Input: part model. Units: mm. Frame: model coordinates. A direction names the side the tool comes from. Round coordinates to 2 decimals unless told otherwise and drop trailing zeros. Loops run counter-clockwise (first coordinate to the right, second up) from the corner with the lowest first, then second, coordinate; pieces in that order, holes last. Notation, with made-up numbers: (65, -14.75) - (109, -14.75) arc R13 ccw to (109, 0.25) - close; hole circle Ø10 at (26.25, 13). An arc over 180 degrees is marked (long way). Use CSV: the item, a comma, the result in double quotes. Start each with the question number.
1. Pin query (flat end, axial travel): P1, Ø5, axis at y = 3.5, z = -101.5, coming from the -X side; P2, Ø2, axis at x = 11, y = 19.5, coming from the -Z side; P3, Ø4, axis at x = 11.5, y = 15.5, coming from the +Z side. Return the tip coordinate at first contact, or that it passes through.
2. Cut plane C-C (z = -21.5). Return loops of the section in (x, y) (3 decimals).
3. Cut plane B-B (z = -69.7). Return loops of the section in (x, y), and give its area (3 significant figures).
4. Access query for faces 1 (the flat face through (0, 9, -13)), 2 (the flat face through (24, 20, -85.5)), 3 (the cylindrical face through (46.55, 5.46, -69.59)), 4 (the flat face through (21.5, 15, -95)), 5 (the flat face through (0, 9, -5)). Directions: +Z, -Z, +X, -X, +Y, -Y. A direction counts if a zero-diameter tool reaches every point of the face in a straight line with its end or side. Return the directions, or none.
5. Cut plane A-A (z = -53). Return loops of the section in (x, y).
6. Pull-direction query (Y, two-part tool) for faces 6 (the flat face through (48.2, 6, -102)), 7 (the flat face through (0, 9, -25)), 8 (the flat face through (54, 11.8, -102)); classes: +Y half, -Y half, draft (parallel to the pull), parting line (faces both ways), or undercut.
7. Material intervals for probe 1 along Z at (x, y) = (24, 21.75); probe 2 along X at (y, z) = (17.5, -88); probe 3 along X at (y, z) = (6.95, -69.7), sorted ascending. Write a range as from..to.
```python
from build123d import *

# Parameters (mm, degrees)
EXTRUDE_1_DEPTH     = 60
SHELL_1_T           = -2.5
SKETCH_3_R          = 2.25
EXTRUDE_3_DEPTH     = 4
CUT_EXTRUDE_1_DEPTH = 118.856904762
SKETCH_5_R          = 2.2
EXTRUDE_4_DEPTH     = 6
SKETCH_7_W          = 42
SKETCH_7_H          = 12
CUT_EXTRUDE_3_DEPTH = 2.5
SKETCH_8_W          = 10.4
SKETCH_8_H          = 12
EXTRUDE_5_DEPTH     = 2.5
SKETCH_9_W          = 7
SKETCH_9_H          = 7
SKETCH_9_R          = 2.2
EXTRUDE_6_DEPTH     = 8
SKETCH_10_R         = 2.2
EXTRUDE_7_DEPTH     = 5
EXTRUDE_8_DEPTH     = 4
EXTRUDE_10_DEPTH    = 4
SKETCH_14_R         = 3
CUT_EXTRUDE_4_DEPTH = 119.584358159
SKETCH_15_W         = 16
SKETCH_15_H         = 2
CUT_EXTRUDE_5_DEPTH = 1.4
CUT_EXTRUDE_6_REACH = 121.933
SKETCH_16_W         = 12
SKETCH_16_H         = 14
SKETCH_17_W         = 12
SKETCH_17_H         = 14
EXTRUDE_14_DEPTH    = 2
EXTRUDE_15_REACH    = 120.238
SKETCH_18_W         = 3.2
SKETCH_18_H         = 3.2
SKETCH_19_W         = 5.75
SKETCH_19_H         = 10.4
CUT_EXTRUDE_7_DEPTH = 4
SKETCH_20_W         = 55
SKETCH_20_H         = 3
CUT_EXTRUDE_8_DEPTH = 0.5
SKETCH_22_R         = 2.2
EXTRUDE_17_DEPTH    = 5
SKETCH_23_R         = 2.897416755
EXTRUDE_18_DEPTH    = 2
FILLET_1_R          = 2
CUT_EXTRUDE_9_REACH = 127.999
SKETCH_25_W         = 5.8
SKETCH_25_H         = 5.8
SKETCH_26_W         = 5.8
SKETCH_26_H         = 4
EXTRUDE_19_DEPTH    = 1
SKETCH_27_W         = 10
SKETCH_27_H         = 4
EXTRUDE_20_DEPTH    = 2
SKETCH_28_W         = 11.8
SKETCH_28_H         = 11.8
SKETCH_28_W_2       = 5.8
SKETCH_28_H_2       = 5.8
EXTRUDE_23_DEPTH    = 4.5


with BuildPart() as part:
    # 草图1 → 凸台-拉伸1 (new body)
    with BuildSketch(Plane(origin=(0, 0, 0), x_dir=(0, 0, -1), z_dir=(1, 0, 0))):
        Polygon((0, 0), (100, 0), (100, 28), (0, 17), align=None)
    extrude(amount=EXTRUDE_1_DEPTH)

    # 抽壳1
    shell_1_openings = [part.faces().sort_by_distance(p)[0] for p in [
        (30, 22.5, -50),
    ]]
    offset(amount=SHELL_1_T, openings=shell_1_openings, kind=Kind.INTERSECTION)

    # 草图3 → 凸台-拉伸3 (add)
    # profile 1 of 2: a face of its own
    with BuildSketch(Plane(origin=(0, 2.5, 0), x_dir=(1, 0, 0), z_dir=(0, 1, 0))):
        with BuildLine():
            Line((2.5, 97.5), (2.5, 85.75))
            ThreePointArc((2.5, 85.75), (6.685854123, 84.442437632), (9.25, 88))
            Line((9.25, 88), (9.25, 97.5))
            Line((9.25, 97.5), (2.5, 97.5))
        make_face()
        with Locations(Location((5.5, 88, 0), (0, 0, 270))):
            Circle(SKETCH_3_R, mode=Mode.SUBTRACT)
    # profile 2 of 2: a face of its own
    with BuildSketch(Plane(origin=(0, 2.5, 0), x_dir=(1, 0, 0), z_dir=(0, 1, 0))):
        with BuildLine():
            Line((16.75, 88), (16.75, 97.5))
            Line((16.75, 97.5), (24.25, 97.5))
            Line((24.25, 97.5), (24.25, 88))
            ThreePointArc((24.25, 88), (20.5, 84.25), (16.75, 88))
        make_face()
        with Locations(Location((20.5, 88, 0), (0, 0, 270))):
            Circle(SKETCH_3_R, mode=Mode.SUBTRACT)
    extrude(amount=EXTRUDE_3_DEPTH)

    # 草图4 → 切除-拉伸1 (cut, through all)
    with BuildSketch(Plane.XY.offset(-97.5)):
        Polygon((17, 8.3), (24.25, 8.3), (24.25, 6.5), (2.5, 6.5), (2.5, 8.3), (9, 8.3), (9, 13), (17, 13), align=None)
    extrude(amount=-CUT_EXTRUDE_1_DEPTH, mode=Mode.SUBTRACT)

    # 草图5 → 凸台-拉伸4 (add)
    # profile 1 of 4: a face of its own
    with BuildSketch(Plane(origin=(0, 2.5, 0), x_dir=(1, 0, 0), z_dir=(0, 1, 0))):
        with BuildLine():
            Line((5.032858412, 2.5), (11.467141588, 2.5))
            ThreePointArc((11.467141588, 2.5), (8.25, 9.4), (5.032858412, 2.5))
        make_face()
        with Locations(Location((8.25, 5.2, 0), (0, 0, 270))):
            Circle(SKETCH_5_R, mode=Mode.SUBTRACT)
    # profile 2 of 4: a face of its own
    with BuildSketch(Plane(origin=(0, 2.5, 0), x_dir=(1, 0, 0), z_dir=(0, 1, 0))):
        with BuildLine():
            Line((48.532858412, 2.5), (54.967141588, 2.5))
            ThreePointArc((54.967141588, 2.5), (51.75, 9.4), (48.532858412, 2.5))
        make_face()
        with Locations(Location((51.75, 5.2, 0), (0, 0, 90))):
            Circle(SKETCH_5_R, mode=Mode.SUBTRACT)
    # profile 3 of 4: a face of its own
    with BuildSketch(Plane(origin=(0, 2.5, 0), x_dir=(1, 0, 0), z_dir=(0, 1, 0))):
        with BuildLine():
            Line((8.25, 74.9), (2.5, 74.9))
            Line((2.5, 74.9), (2.5, 64.5))
            Line((2.5, 64.5), (8.25, 64.5))
            ThreePointArc((8.25, 64.5), (13.45, 69.7), (8.25, 74.9))
        make_face()
        with Locations(Location((8.25, 69.7, 0), (0, 0, 270))):
            Circle(SKETCH_5_R, mode=Mode.SUBTRACT)
    # profile 4 of 4: a face of its own
    with BuildSketch(Plane(origin=(0, 2.5, 0), x_dir=(1, 0, 0), z_dir=(0, 1, 0))):
        with BuildLine():
            Line((51.75, 74.9), (57.5, 74.9))
            Line((57.5, 74.9), (57.5, 64.5))
            Line((57.5, 64.5), (51.75, 64.5))
            ThreePointArc((51.75, 64.5), (46.55, 69.7), (51.75, 74.9))
        make_face()
        with Locations(Location((51.75, 69.7, 0), (0, 0, 90))):
            Circle(SKETCH_5_R, mode=Mode.SUBTRACT)
    extrude(amount=EXTRUDE_4_DEPTH)

    # 草图7 → 切除-拉伸3 (cut)
    with BuildSketch(Plane(origin=(60, 0, 0), x_dir=(0, 0, -1), z_dir=(1, 0, 0))):
        with Locations((69, 6)):
            Rectangle(SKETCH_7_W, SKETCH_7_H)
    extrude(amount=-CUT_EXTRUDE_3_DEPTH, mode=Mode.SUBTRACT)

    # 草图8 → 凸台-拉伸5 (add)
    with BuildSketch(Plane(origin=(57.5, 0, 0), x_dir=(0, 0, -1), z_dir=(1, 0, 0))):
        with Locations((69.7, 6)):
            Rectangle(SKETCH_8_W, SKETCH_8_H)
    extrude(amount=EXTRUDE_5_DEPTH)

    # 草图9 → 凸台-拉伸6 (add)
    with BuildSketch(Plane(origin=(0, 18, 0), x_dir=(1, 0, 0), z_dir=(0, 1, 0))):
        with Locations((6, 94)):
            Rectangle(SKETCH_9_W, SKETCH_9_H)
        with Locations(Location((6, 94, 0), (0, 0, 270))):
            Circle(SKETCH_9_R, mode=Mode.SUBTRACT)
    extrude_6 = extrude(amount=EXTRUDE_6_DEPTH)

    # 草图10 → 凸台-拉伸7 (add)
    with BuildSketch(Plane.XZ.offset(-18)):
        with Locations(Location((6, -94, 0), (0, 0, 270))):
            Circle(SKETCH_10_R)
    extrude(amount=-EXTRUDE_7_DEPTH)

    # 草图11 → 凸台-拉伸8 (add)
    with BuildSketch(Plane.XZ.offset(-18)):
        Polygon((9.5, -97.5), (25.5, -97.5), (25.5, -91.9), (23.5, -91.9), (23.5, -89.9), (25.5, -89.9), (25.5, -85.5), (9.5, -85.5), (9.5, -89.9), (11.5, -89.9), (11.5, -91.9), (9.5, -91.9), align=None)
    extrude(amount=-EXTRUDE_8_DEPTH)

    # 草图13 → 凸台-拉伸10 (add)
    with BuildSketch(Plane(origin=(25.5, 0, 0), x_dir=(0, 0, -1), z_dir=(1, 0, 0))):
        Polygon((85.5, 18), (97.5, 11), (97.5, 18), align=None)
    extrude(amount=-EXTRUDE_10_DEPTH)

    # 草图14 → 切除-拉伸4 (cut, through all)
    with BuildSketch(Plane(origin=(0, 6.5, 0), x_dir=(1, 0, 0), z_dir=(0, 1, 0))):
        with Locations((20.5, 88)):
            Circle(SKETCH_14_R)
    extrude(amount=CUT_EXTRUDE_4_DEPTH, mode=Mode.SUBTRACT)

    # 草图15 → 切除-拉伸5 (cut)
    with BuildSketch(Plane(origin=(0, 22, 0), x_dir=(1, 0, 0), z_dir=(0, 1, 0))):
        with Locations((17.5, 96.5)):
            Rectangle(SKETCH_15_W, SKETCH_15_H)
    extrude(amount=-CUT_EXTRUDE_5_DEPTH, mode=Mode.SUBTRACT)

    # 镜向2: 凸台-拉伸6 across plane
    add(extrude_6.mirror(Plane.ZY.offset(-30)))

    # 草图16 → 切除-拉伸6 (cut, up to next)
    with BuildSketch(Plane.ZY, mode=Mode.PRIVATE) as cut_extrude_6_sk1:
        with Locations((-19, 9.5)):
            Rectangle(SKETCH_16_W, SKETCH_16_H)
    cut_extrude_6_tool1 = extrude(cut_extrude_6_sk1.sketch, amount=-CUT_EXTRUDE_6_REACH, mode=Mode.PRIVATE) & part.part
    add(cut_extrude_6_tool1.solids().sort_by_distance((0, 9.5, -19))[0], mode=Mode.SUBTRACT)

    # 草图17 → 凸台-拉伸14 (add)
    with BuildSketch(Plane.ZY):
        Polygon((-27.5, 0), (-10.5, 0), (-10.5, 18.155), (-18.181818182, 19), (-27.5, 19), align=None)
        with Locations((-19, 9.5)):
            Rectangle(SKETCH_17_W, SKETCH_17_H, mode=Mode.SUBTRACT)
    extrude(amount=EXTRUDE_14_DEPTH)

    # 凸台-拉伸15: up to this plane
    extrude_15_end = Plane(origin=(60, 25.51498911, -100.273351198), z_dir=(0, -0.9940043559354329, -0.10934047915289762))
    # 草图18 → 凸台-拉伸15 (add, up to the surface)
    with BuildSketch(Plane(origin=(0, 8.5, 0), x_dir=(1, 0, 0), z_dir=(0, 1, 0)), mode=Mode.PRIVATE) as extrude_15_sk1:
        with Locations((55.9, 73.3)):
            Rectangle(SKETCH_18_W, SKETCH_18_H)
    extrude_15_tool1 = split(extrude(extrude_15_sk1.sketch, amount=EXTRUDE_15_REACH, mode=Mode.PRIVATE), bisect_by=extrude_15_end, keep=Keep.BOTH, mode=Mode.PRIVATE)
    add(extrude_15_tool1.solids().sort_by_distance((55.9, 8.5, -73.3))[0])
    # 草图18 → 凸台-拉伸15 (add, up to the surface)
    with BuildSketch(Plane(origin=(0, 8.5, 0), x_dir=(1, 0, 0), z_dir=(0, 1, 0)), mode=Mode.PRIVATE) as extrude_15_sk2:
        with Locations((55.9, 66.1)):
            Rectangle(SKETCH_18_W, SKETCH_18_H)
    extrude_15_tool2 = split(extrude(extrude_15_sk2.sketch, amount=EXTRUDE_15_REACH, mode=Mode.PRIVATE), bisect_by=extrude_15_end, keep=Keep.BOTH, mode=Mode.PRIVATE)
    add(extrude_15_tool2.solids().sort_by_distance((55.9, 8.5, -66.1))[0])

    # 草图19 → 切除-拉伸7 (cut)
    with BuildSketch(Plane(origin=(0, 8.5, 0), x_dir=(1, 0, 0), z_dir=(0, 1, 0))):
        with Locations((54.625, 69.7)):
            Rectangle(SKETCH_19_W, SKETCH_19_H)
    extrude(amount=CUT_EXTRUDE_7_DEPTH, mode=Mode.SUBTRACT)

    # 草图20 → 切除-拉伸8 (cut)
    with BuildSketch(Plane(origin=(0, 0, -2.5), x_dir=(-1, 0, 0), z_dir=(0, 0, -1))):
        with Locations((-30, 10)):
            Rectangle(SKETCH_20_W, SKETCH_20_H)
    extrude(amount=-CUT_EXTRUDE_8_DEPTH, mode=Mode.SUBTRACT)

    # 草图22 → 凸台-拉伸17 (add)
    with BuildSketch(Plane(origin=(0, 17, 0), x_dir=(1, 0, 0), z_dir=(0, 1, 0))):
        with BuildLine():
            Line((25.3, -2.5), (25.3, 0))
            Line((25.3, 0), (34.7, 0))
            Line((34.7, 0), (34.7, -2.5))
            ThreePointArc((34.7, -2.5), (30, -7.2), (25.3, -2.5))
        make_face()
        with Locations(Location((30, -2.5, 0), (0, 0, 270))):
            Circle(SKETCH_22_R, mode=Mode.SUBTRACT)
    extrude(amount=-EXTRUDE_17_DEPTH)

    # 草图23 → 凸台-拉伸18 (add)
    with BuildSketch(Plane.XZ.offset(-12)):
        with Locations((30, 2.5)):
            Circle(SKETCH_23_R)
    extrude(amount=-EXTRUDE_18_DEPTH)

    # 圆角1
    fillet_1_edges = [part.edges().sort_by_distance(p)[0] for p in [
        (30, 12, 7.2),
        (25.3, 12, 1.25),
        (30, 12, 0),
        (25.3, 14.5, 0),
        (34.7, 12, 1.25),
        (34.7, 14.5, 0),
    ]]
    fillet(fillet_1_edges, radius=FILLET_1_R)

    # 草图25 → 切除-拉伸9 (cut, up to next)
    with BuildSketch(Plane(origin=(0, 0, -100), x_dir=(-1, 0, 0), z_dir=(0, 0, -1)), mode=Mode.PRIVATE) as cut_extrude_9_sk1:
        with Locations((-54.1, 5.9)):
            Rectangle(SKETCH_25_W, SKETCH_25_H)
    cut_extrude_9_tool1 = extrude(cut_extrude_9_sk1.sketch, amount=-CUT_EXTRUDE_9_REACH, mode=Mode.PRIVATE) & part.part
    add(cut_extrude_9_tool1.solids().sort_by_distance((54.1, 5.9, -100))[0], mode=Mode.SUBTRACT)

    # 草图26 → 凸台-拉伸19 (add)
    with BuildSketch(Plane.XY.offset(-97.5)):
        with Locations((54.1, 5.9)):
            Rectangle(SKETCH_26_W, SKETCH_26_H)
    extrude(amount=-EXTRUDE_19_DEPTH)

    # 草图27 → 凸台-拉伸20 (add)
    with BuildSketch(Plane.XY.offset(-97.5)):
        with Locations((54.1, 5.9)):
            Rectangle(SKETCH_27_W, SKETCH_27_H)
    extrude(amount=EXTRUDE_20_DEPTH)

    # 草图28 → 凸台-拉伸23 (add)
    with BuildSketch(Plane(origin=(0, 0, -100), x_dir=(-1, 0, 0), z_dir=(0, 0, -1))):
        with Locations((-54.1, 5.9)):
            Rectangle(SKETCH_28_W, SKETCH_28_H)
        with Locations((-54.1, 5.9)):
            Rectangle(SKETCH_28_W_2, SKETCH_28_H_2, mode=Mode.SUBTRACT)
    extrude(amount=EXTRUDE_23_DEPTH)


solid = part.part
```
Established:
1,P1,"stops at x = 0"
1,P2,"stops at z = -100"
1,P3,"stops at z = 0"
2,outline,"(-2, 0) - (60, 0) - (60, 19.365) - (57.5, 19.365) - (57.5, 2.5) - (-2, 2.5) - close; (-2, 16.5) - (2.5, 16.5) - (2.5, 19.365) - (0, 19.365) - (0, 19) - (-2, 19) - close"
3,outline,"(0, 0) - (60, 0) - (60, 24.67) - (57.5, 24.67) - (57.5, 8.5) - (53.95, 8.5) - (53.95, 2.5) - (49.55, 2.5) - (49.55, 8.5) - (46.55, 8.5) - (46.55, 2.5) - (13.45, 2.5) - (13.45, 8.5) - (10.45, 8.5) - (10.45, 2.5) - (6.05, 2.5) - (6.05, 8.5) - (2.5, 8.5) - (2.5, 24.67) - (0, 24.67) - close"
3,area,"339 mm2"
4,face 1,"-X"
4,face 2,"+Z, +Y"
4,face 3,"+Y"
4,face 4,"none"
4,face 5,"+Z, -X, +Y, -Y"
5,outline,"(0, 0) - (57.5, 0) - (57.5, 2.5) - (2.5, 2.5) - (2.5, 22.83) - (0, 22.83) - close; (57.5, 12) - (60, 12) - (60, 22.83) - (57.5, 22.83) - close"
6,face 6,"draft"
6,face 7,"undercut"
6,face 8,"+Y half"
7,probe 1,"z = -100..-97.5, -95.5..-91.9, -89.9..-85.5"
7,probe 2,"x = 0..2.5, 23.5..25.5, 57.5..60"
7,probe 3,"x = 0..6.05, 10.45..13.45, 46.55..49.55, 53.95..60"
